Input: part model. Units: mm. Frame: model coordinates. Face numbers are marked on the shaded views. A direction names the side the tool comes from. Coordinates: 2 decimals unless noted, no trailing zeros. Order: outer loops, then holes, each group sorted by start corner. A loop starts at its lowest first (then second) coordinate and runs counter-clockwise, first axis right, second up. Notation, with made-up numbers: (41.25, 63) - (96.25, 63) arc R7 cw to (96.25, 72) - close; hole circle Ø7 at (-28.5, 40.5). An arc over 180 degrees is marked (long way). Answer as CSV lines item,"result". Start each with the question number.
Item 1: First-contact query: pin 1 (10 mm diameter, centred on x = 32.5, y = -12.5, fed in from +Z); pin 2 (3.5 mm diameter, centred on x = 53, z = 0, fed in from +Y); pin 3 (1.5 mm diameter, centred on x = -11, z = 36, fed in from +Y); pin 4 (3 mm diameter, centred on x = -30, y = -19.5, fed in from -Z). Flat tips, straight axial feed; report the tip coordinate or a pass-through.
Item 2: Section D-D (z = 53). Output: boundary loops of the cut face in (x, y).
Item 3: Material intervals for line 1 along Z through (x, y) = (0, -47.25); line 2 along X through (y, z) = (-31, 0); line 3 along Z through (x, y) = (0, -2.7), sorted ascending.
Item 4: Access query for the marked faces 4, 5, 6 and 7. Directions: +Z, -Z, +X, -X, +Y, -Y. A direction counts if a zero-diameter tool reaches every point of the face in a straight line with its end or side. Return the directions, or none.
Item 5: Draft query along Z for the marked faces 1, 2 and 3. Return one class per face: +Z half, -Z half, draft (parallel to the pull), parting line (faces both ways), or undercut.
Item 6: Section B-B (x = 0). State how many separate pieces and enclosed holes the cut face has, and give its area (3 significant figures).
Item 7: Section A-A (y = -13). Output: boundary loops of the cut face in (x, z).
from build123d import *

# Parameters (mm, degrees)
SKETCH1_R                  = 60
STOCK_DEPTH                = 50
HOLLOWINTERIOR_REACH       = 57
HOLLOWINTERIOR_START       = -5
SKETCH8_R                  = 35
SKETCH7_R                  = 10.5
HOLEFORMOTORSHAFT_DEPTH    = 51
SKETCH9_OUTSIDE_W          = 157.384
SKETCH9_OUTSIDE_H          = 157.384
SKETCH9_OUTSIDE_R          = 37.5
EXTERIORLATHE_DEPTH        = 45
CHAMFER1_SIZE              = 10
CHAMFER2_SIZE              = 10
CHAMFER3_SIZE              = 10
SLOTSFORFUN_DEPTH          = 45
SKETCH13_R                 = 2
GEARBOXMOUNTINGHOLES_DEPTH = 5
CUT_EXTRUDE5_START         = -45
SKETCH14_R                 = 3
CUT_EXTRUDE5_DEPTH         = 5


with BuildPart() as part:
    # Sketch1 → Stock (new body)
    with BuildSketch(Plane(origin=(0, 0, 0), x_dir=(1, 0, 0), z_dir=(0, 1, 0))):
        Circle(SKETCH1_R)
    extrude(amount=-STOCK_DEPTH)

    # Sketch8 → HollowInterior (cut, up to next)
    with BuildSketch(Plane(origin=(0, 0, 0), x_dir=(1, 0, 0), z_dir=(0, 1, 0)).offset(HOLLOWINTERIOR_START), mode=Mode.PRIVATE) as hollowinterior_sk1:
        Circle(SKETCH8_R)
    hollowinterior_tool1 = extrude(hollowinterior_sk1.sketch, amount=-HOLLOWINTERIOR_REACH, mode=Mode.PRIVATE) & part.part
    add(hollowinterior_tool1.solids().sort_by_distance((0, -5, 0))[0], mode=Mode.SUBTRACT)

    # Sketch7 → HoleForMotorShaft (cut, through all)
    with BuildSketch(Plane(origin=(0, 0, 0), x_dir=(1, 0, 0), z_dir=(0, 1, 0))):
        Circle(SKETCH7_R)
    extrude(amount=-HOLEFORMOTORSHAFT_DEPTH, mode=Mode.SUBTRACT)

    # Sketch9 outside → ExteriorLathe (cut)
    with BuildSketch(Plane(origin=(0, 0, 0), x_dir=(1, 0, 0), z_dir=(0, 1, 0))):
        Rectangle(SKETCH9_OUTSIDE_W, SKETCH9_OUTSIDE_H)
        Circle(SKETCH9_OUTSIDE_R, mode=Mode.SUBTRACT)
    extrude(amount=-EXTERIORLATHE_DEPTH, mode=Mode.SUBTRACT)

    # Chamfer1
    chamfer1_edges = [part.edges().sort_by_distance(p)[0] for p in [
        (-35, -5, 0),
    ]]
    chamfer(chamfer1_edges, length=CHAMFER1_SIZE)

    # Chamfer2
    chamfer2_edges = [part.edges().sort_by_distance(p)[0] for p in [
        (-37.5, 0, 0),
    ]]
    chamfer(chamfer2_edges, length=CHAMFER2_SIZE)

    # Chamfer3
    chamfer3_edges = [part.edges().sort_by_distance(p)[0] for p in [
        (-37.5, -45, 0),
    ]]
    chamfer(chamfer3_edges, length=CHAMFER3_SIZE)

    # Sketch10 → SlotsForFun (cut)
    with BuildSketch(Plane(origin=(0, 0, 0), x_dir=(1, 0, 0), z_dir=(0, 1, 0))):
        Polygon((-10.606601718, 17.67766953), (-30.0520382, 37.123106012), (-37.123106012, 30.0520382), (-17.67766953, 10.606601718), align=None)
        Polygon((17.67766953, 10.606601718), (37.123106012, 30.0520382), (30.0520382, 37.123106012), (10.606601718, 17.67766953), align=None)
        Polygon((10.606601718, -17.67766953), (30.0520382, -37.123106012), (37.123106012, -30.0520382), (17.67766953, -10.606601718), align=None)
        Polygon((-17.67766953, -10.606601718), (-37.123106012, -30.0520382), (-30.0520382, -37.123106012), (-10.606601718, -17.67766953), align=None)
    extrude(amount=-SLOTSFORFUN_DEPTH, mode=Mode.SUBTRACT)

    # Sketch13 → GearboxMountingHoles (cut)
    with BuildSketch(Plane(origin=(0, 0, 0), x_dir=(1, 0, 0), z_dir=(0, 1, 0))):
        with Locations((0, 17.5)):
            Circle(SKETCH13_R)
        with Locations((17.5, 0)):
            Circle(SKETCH13_R)
        with Locations((0, -17.5)):
            Circle(SKETCH13_R)
        with Locations((-17.5, 0)):
            Circle(SKETCH13_R)
    extrude(amount=-GEARBOXMOUNTINGHOLES_DEPTH, mode=Mode.SUBTRACT)

    # Sketch14 → Cut-Extrude5 (cut)
    with BuildSketch(Plane(origin=(0, 0, 0), x_dir=(1, 0, 0), z_dir=(0, 1, 0)).offset(CUT_EXTRUDE5_START)):
        with Locations((0, 53)):
            Circle(SKETCH14_R)
        with Locations((53, 0)):
            Circle(SKETCH14_R)
        with Locations((0, -53)):
            Circle(SKETCH14_R)
        with Locations((-53, 0)):
            Circle(SKETCH14_R)
    extrude(amount=-CUT_EXTRUDE5_DEPTH, mode=Mode.SUBTRACT)


solid = part.part
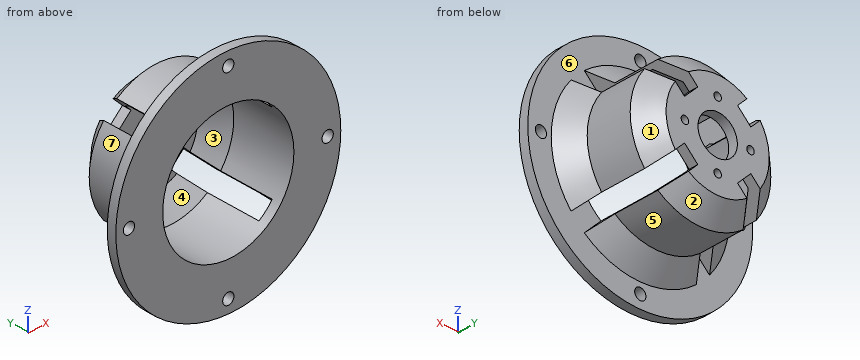
Determined:
1,pin 1,"stops at z = 22.74"
1,pin 2,"passes through"
1,pin 3,"stops at y = -9.39"
1,pin 4,"stops at z = -22.74"
2,outline,"(-28.12, -50) - (-3, -50) - (-3, -45) - (-28.12, -45) - close; (3, -50) - (28.12, -50) - (28.12, -45) - (3, -45) - close"
3,line 1,"z = -60 to -56, -50 to -35, 35 to 50, 56 to 60"
3,line 2,"x = -37.5 to -35, 35 to 37.5"
3,line 3,"z = -30.2 to -19.5, -15.5 to -10.5, 10.5 to 15.5, 19.5 to 30.2"
4,face 4,"-Y"
4,face 5,"-Z, +Y"
4,face 6,"+Y"
4,face 7,"-X, +Y"
5,face 1,"parting line"
5,face 2,"-Z half"
5,face 3,"undercut"
6,separate pieces,"6"
6,enclosed holes,"0"
6,area,"720 mm^2"
7,outline,"(-29.82, -22.74) - (-26.6, -19.53) arc R33 cw to (-26.6, 19.53) - (-29.82, 22.74) arc R37.5 ccw to start; (-22.74, -29.82) arc R37.5 ccw to (22.74, -29.82) - (19.53, -26.6) arc R33 cw to (-19.53, -26.6) - close; (-22.74, 29.82) - (-19.53, 26.6) arc R33 cw to (19.53, 26.6) - (22.74, 29.82) arc R37.5 ccw to start; (26.6, -19.53) - (29.82, -22.74) arc R37.5 ccw to (29.82, 22.74) - (26.6, 19.53) arc R33 cw to start"
